Build history of the part. All positions in model axes, mm. A direction names the side the tool comes from. Give positions to 0.01 mm unless a question says otherwise; leave off trailing zeros. Write each loop counter-clockwise with the first axis right and the second up, starting at its lowest first coordinate (ties: lowest second). Pieces come first, ordered by that corner, then holes. Notation, with made-up numbers: (56, 32) -> (68, 32) arc R17 ccw to (68, 42) -> close; hole circle Ø8 at (-10.5, 46.25). An arc over 180 degrees is marked (long way). Put each result on its own line as item: value. Start each with the question number.
Item 1: Slice it at B-B, the plane z = -71.8. List the corners of the cut face in (x, y).
Item 2: Flat gauge pins, fed straight in: pin 1 Ø16 at (x, z) = (0, 0) entering from +Y; pin 2 Ø6 at (x, y) = (-44, 4) entering from +Z; pin 3 Ø8 at (x, z) = (51.96, -30) entering from +Y; pin 4 Ø5 at (x, z) = (57.96, 15.53) entering from +Y. Where does each tip first touch, or does it go through?
Item 3: Tool access for faces 1 (the cylindrical face through (3.604, 2.465, -11.446)), 2 (the flat face through (-15, 3, -58)): list every direction of +Z, -Z, +X, -X, +Y, -Y with a clear straight run to the whole face (end or side of a thin tool).
Item 4: Drill centre lines: line 1 along Z through (x, y) = (1, 13.25); line 2 along X through (y, z) = (4.55, 30); line 3 along Z through (x, y) = (2, 5.25). Where is each one in solid material? Low to high.
Item 5: Slice it at C-C, the plane y = 19.5. Give the number of separate pieces and of enclosed holes in the cut face, plus the area to 3 significant figures.
Item 6: Slice it at D-D, the plane x = -30. List the corners of the cut face in (y, z).
```python
from build123d import *

# Parameters (mm, degrees)
SKETCH1_R           = 77.1
BOSS_EXTRUDE1_DEPTH = 24.6
SKETCH2_R           = 67
CUT_EXTRUDE1_DEPTH  = 16.6
SKETCH3_R           = 3
CUT_EXTRUDE2_DEPTH  = 5
SKETCH4_R           = 12
CUT_EXTRUDE3_DEPTH  = 5
SKETCH5_R           = 9
CUT_EXTRUDE4_DEPTH  = 5
SKETCH6_R           = 2.8
CUT_EXTRUDE5_DEPTH  = 8


with BuildPart() as part:
    # Sketch1 → Boss-Extrude1 (new body)
    with BuildSketch(Plane(origin=(0, 0, 0), x_dir=(1, 0, 0), z_dir=(0, 1, 0))):
        with Locations(Location((0, 0, 0), (0, 0, 270))):
            Circle(SKETCH1_R)
    extrude(amount=BOSS_EXTRUDE1_DEPTH)

    # Sketch2 → Cut-Extrude1 (cut)
    with BuildSketch(Plane(origin=(0, 24.6, 0), x_dir=(1, 0, 0), z_dir=(0, 1, 0))):
        with Locations(Location((0, 0, 0), (0, 0, 270))):
            Circle(SKETCH2_R)
    extrude(amount=-CUT_EXTRUDE1_DEPTH, mode=Mode.SUBTRACT)

    # Sketch3 → Cut-Extrude2 (cut)
    with BuildSketch(Plane(origin=(0, 8, 0), x_dir=(1, 0, 0), z_dir=(0, 1, 0))):
        with Locations(Location((60, 0, 0), (0, 0, 270))):
            Circle(SKETCH3_R)
        with Locations(Location((57.955549577, -15.529142706, 0), (0, 0, 270))):
            Circle(SKETCH3_R)
        with Locations(Location((51.961524227, -30, 0), (0, 0, 270))):
            Circle(SKETCH3_R)
        with Locations(Location((42.426406871, -42.426406871, 0), (0, 0, 270))):
            Circle(SKETCH3_R)
        with Locations(Location((30, -51.961524227, 0), (0, 0, 270))):
            Circle(SKETCH3_R)
        with Locations(Location((15.529142706, -57.955549577, 0), (0, 0, 270))):
            Circle(SKETCH3_R)
        with Locations(Location((0, -60, 0), (0, 0, 270))):
            Circle(SKETCH3_R)
        with Locations(Location((-15.529142706, -57.955549577, 0), (0, 0, 270))):
            Circle(SKETCH3_R)
        with Locations(Location((-30, -51.961524227, 0), (0, 0, 270))):
            Circle(SKETCH3_R)
        with Locations(Location((-42.426406871, -42.426406871, 0), (0, 0, 270))):
            Circle(SKETCH3_R)
        with Locations(Location((-51.961524227, -30, 0), (0, 0, 270))):
            Circle(SKETCH3_R)
        with Locations(Location((-57.955549577, -15.529142706, 0), (0, 0, 270))):
            Circle(SKETCH3_R)
        with Locations(Location((-60, 0, 0), (0, 0, 270))):
            Circle(SKETCH3_R)
        with Locations(Location((-57.955549577, 15.529142706, 0), (0, 0, 270))):
            Circle(SKETCH3_R)
        with Locations(Location((-51.961524227, 30, 0), (0, 0, 270))):
            Circle(SKETCH3_R)
        with Locations(Location((-42.426406871, 42.426406871, 0), (0, 0, 270))):
            Circle(SKETCH3_R)
        with Locations(Location((-30, 51.961524227, 0), (0, 0, 270))):
            Circle(SKETCH3_R)
        with Locations(Location((-15.529142706, 57.955549577, 0), (0, 0, 270))):
            Circle(SKETCH3_R)
        with Locations(Location((0, 60, 0), (0, 0, 270))):
            Circle(SKETCH3_R)
        with Locations(Location((15.529142706, 57.955549577, 0), (0, 0, 270))):
            Circle(SKETCH3_R)
        with Locations(Location((30, 51.961524227, 0), (0, 0, 270))):
            Circle(SKETCH3_R)
        with Locations(Location((42.426406871, 42.426406871, 0), (0, 0, 270))):
            Circle(SKETCH3_R)
        with Locations(Location((51.961524227, 30, 0), (0, 0, 270))):
            Circle(SKETCH3_R)
        with Locations(Location((57.955549577, 15.529142706, 0), (0, 0, 270))):
            Circle(SKETCH3_R)
    extrude(amount=-CUT_EXTRUDE2_DEPTH, mode=Mode.SUBTRACT)

    # Sketch4 → Cut-Extrude3 (cut)
    with BuildSketch(Plane.XZ):
        with Locations(Location((0, 0, 0), (0, 0, 270))):
            Circle(SKETCH4_R)
    extrude(amount=-CUT_EXTRUDE3_DEPTH, mode=Mode.SUBTRACT)

    # Sketch5 → Cut-Extrude4 (cut)
    with BuildSketch(Plane(origin=(0, 8, 0), x_dir=(1, 0, 0), z_dir=(0, 1, 0))):
        with Locations(Location((0, 0, 0), (0, 0, 270))):
            Circle(SKETCH5_R)
    extrude(amount=-CUT_EXTRUDE4_DEPTH, mode=Mode.SUBTRACT)

    # Sketch6 → Cut-Extrude5 (cut)
    with BuildSketch(Plane(origin=(0, 24.6, 0), x_dir=(1, 0, 0), z_dir=(0, 1, 0))):
        with Locations(Location((0, 71.8, 0), (0, 0, 270))):
            Circle(SKETCH6_R)
        with Locations(Location((50.770266889, 50.770266889, 0), (0, 0, 270))):
            Circle(SKETCH6_R)
        with Locations(Location((71.8, 0, 0), (0, 0, 270))):
            Circle(SKETCH6_R)
        with Locations(Location((50.770266889, -50.770266889, 0), (0, 0, 270))):
            Circle(SKETCH6_R)
        with Locations(Location((0, -71.8, 0), (0, 0, 270))):
            Circle(SKETCH6_R)
        with Locations(Location((-50.770266889, -50.770266889, 0), (0, 0, 270))):
            Circle(SKETCH6_R)
        with Locations(Location((-71.8, 0, 0), (0, 0, 270))):
            Circle(SKETCH6_R)
        with Locations(Location((-50.770266889, 50.770266889, 0), (0, 0, 270))):
            Circle(SKETCH6_R)
    extrude(amount=-CUT_EXTRUDE5_DEPTH, mode=Mode.SUBTRACT)


solid = part.part
```
Values follow:
1. outline: (-28.09, 0) -> (28.09, 0) -> (28.09, 24.6) -> (2.8, 24.6) -> (2.8, 16.6) -> (-2.8, 16.6) -> (-2.8, 24.6) -> (-28.09, 24.6) -> close
2. pin 1: through
2. pin 2: z = 65.29
2. pin 3: y = 8
2. pin 4: y = 3
3. face 1: -Y
3. face 2: +Y
4. line 1: -77.09 to -66.99, 66.99 to 77.09
4. line 2: -71.02 to -54.96, -48.96 to 48.96, 54.96 to 71.02
4. line 3: -77.07 to -62.24, -57.76 to -8.77, 8.77 to 57.76, 62.24 to 77.07
5. separate pieces: 1
5. enclosed holes: 9
5. area: 4,380 mm2
6. outline: (0, -71.02) -> (24.6, -71.02) -> (24.6, -59.91) -> (8, -59.91) -> (8, -54.96) -> (3, -54.96) -> (3, -48.96) -> (8, -48.96) -> (8, 48.96) -> (3, 48.96) -> (3, 54.96) -> (8, 54.96) -> (8, 59.91) -> (24.6, 59.91) -> (24.6, 71.02) -> (0, 71.02) -> close
